from build123d import *

# Parameters (mm, degrees)
SKETCH1_W           = 128.5875
SKETCH1_H           = 111.125
BOSS_EXTRUDE1_DEPTH = 3.175
SKETCH2_R           = 22.356171926
SKETCH2_R_2         = 6.377074628
SKETCH2_R_3         = 4.503964563
CUT_EXTRUDE1_DEPTH  = 0.508
SKETCH4_R           = 2.446965281
SKETCH4_R_2         = 2.441870248
SKETCH4_R_3         = 1.365573368
SKETCH4_R_4         = 1.359710966
SKETCH4_W           = 6.35
SKETCH4_H           = 2.432656747
SKETCH4_H_2         = 2.571304572
SKETCH4_H_3         = 2.507941143
SKETCH4_H_4         = 2.659157088
CUT_EXTRUDE11_DEPTH = 1.5875


with BuildPart() as part:
    # Sketch1 → Boss-Extrude1 (new body)
    with BuildSketch(Plane(origin=(0, 0, 0), x_dir=(1, 0, 0), z_dir=(0, 1, 0))):
        Rectangle(SKETCH1_W, SKETCH1_H)
    extrude(amount=BOSS_EXTRUDE1_DEPTH)

    # Sketch2 → Cut-Extrude1 (cut)
    # profile 1 of 4: a face of its own
    with BuildSketch(Plane(origin=(0, 3.175, 0), x_dir=(1, 0, 0), z_dir=(0, 1, 0))):
        with BuildLine():
            add(Edge.make_bspline(
                [(-40.987833639, 33.604755502), (-52.791869615, 51.393160856), (-34.670548488, 41.369579914)],
                knots=[0, 0, 0, 1, 1, 1], degree=2))
            ThreePointArc((-40.987833639, 33.604755502), (-38.269367043, 37.845284908), (-34.670548488, 41.369579914))
        make_face()
    # profile 2 of 4: a face of its own
    with BuildSketch(Plane(origin=(0, 3.175, 0), x_dir=(1, 0, 0), z_dir=(0, 1, 0))):
        with BuildLine():
            add(Edge.make_bspline(
                [(-7.184604133, 41.369579914), (7.863520936, 53.974007146), (-0.867318981, 33.604755502)],
                knots=[0, 0, 0, 1, 1, 1], degree=2))
            ThreePointArc((-7.184604133, 41.369579914), (-3.585785578, 37.845284908), (-0.867318981, 33.604755502))
        make_face()
    # profile 3 of 4: a face of its own
    with BuildSketch(Plane(origin=(0, 3.175, 0), x_dir=(1, 0, 0), z_dir=(0, 1, 0))):
        with Locations((-20.92757631, 23.736397022)):
            Circle(SKETCH2_R)
        with Locations(Location((-20.92757631, 17.39779757, 0), (0, 0, 270))):
            Circle(SKETCH2_R_2, mode=Mode.SUBTRACT)
        with Locations(Location((-30.749586512, 27.886542178, 0), (0, 0, 270))):
            Circle(SKETCH2_R_3, mode=Mode.SUBTRACT)
        with Locations(Location((-11.797256967, 27.886542178, 0), (0, 0, 270))):
            Circle(SKETCH2_R_3, mode=Mode.SUBTRACT)
        with BuildLine():
            ThreePointArc((-30.749586512, 9.317085534), (-21.427716956, 3.728530924), (-11.797256967, 8.766728526))
            Line((-11.797256967, 8.766728526), (-30.749586512, 9.317085534))
        make_face(mode=Mode.SUBTRACT)
    # profile 4 of 4: a face of its own
    with BuildSketch(Plane(origin=(0, 3.175, 0), x_dir=(1, 0, 0), z_dir=(0, 1, 0))):
        with BuildLine():
            Line((-11.466221212, -23.168163392), (-10.968659983, -38.249198381))
            Line((-10.968659983, -38.249198381), (-4.570137716, -38.249198381))
            Line((-4.570137716, -38.249198381), (-4.570137716, -29.496558138))
            ThreePointArc((-4.570137716, -29.496558138), (-3.428830963, -30.22282284), (-2.256517086, -30.897894461))
            Line((-2.256517086, -30.897894461), (-1.884638787, -42.169491419))
            Line((-1.884638787, -42.169491419), (4.518768835, -42.169491419))
            Line((4.518768835, -42.169491419), (4.518768835, -33.609716863))
            ThreePointArc((4.518768835, -33.609716863), (14.659430985, -34.563354284), (24.550701184, -32.133286996))
            Line((24.550701184, -32.133286996), (24.780651804, -39.103069122))
            Line((24.780651804, -39.103069122), (31.179561384, -39.103069122))
            Line((31.179561384, -39.103069122), (31.179561384, -28.20870534))
            ThreePointArc((31.179561384, -28.20870534), (32.167865558, -27.406768429), (33.121940536, -26.564397437))
            Line((33.121940536, -26.564397437), (33.604851579, -41.201386667))
            Line((33.604851579, -41.201386667), (40.008784891, -41.201386667))
            Line((40.008784891, -41.201386667), (40.008784891, -17.235252664))
            ThreePointArc((40.008784891, -17.235252664), (34.852114754, 16.699623637), (1.416829228, 24.461630995))
            ThreePointArc((1.416829228, 24.461630995), (1.425653826, 24.099061731), (1.428595616, 23.736397022))
            ThreePointArc((1.428595616, 23.736397022), (-3.993475132, 9.140690788), (-17.629643976, 1.624814864))
            ThreePointArc((-17.629643976, 1.624814864), (-17.261411086, -11.446232799), (-11.466221212, -23.168163392))
        make_face()
    extrude(amount=-CUT_EXTRUDE1_DEPTH, mode=Mode.SUBTRACT)

    # Sketch4 → Cut-Extrude11 (cut)
    with BuildSketch(Plane(origin=(0, 3.175, 0), x_dir=(1, 0, 0), z_dir=(0, 1, 0))):
        with Locations(Location((-30.774197511, 25.825339041, 0), (0, 0, 270))):
            Circle(SKETCH4_R)
        with Locations(Location((-11.798514882, 25.825339041, 0), (0, 0, 270))):
            Circle(SKETCH4_R_2)
        with Locations(Location((-18.425247422, 17.392416095, 0), (0, 0, 270))):
            Circle(SKETCH4_R_3)
        with Locations(Location((-23.55125419, 17.392416095, 0), (0, 0, 270))):
            Circle(SKETCH4_R_4)
        with Locations((-7.793659983, -39.465526755)):
            Rectangle(SKETCH4_W, SKETCH4_H)
        with Locations((1.290361213, -43.455143705)):
            Rectangle(SKETCH4_W, SKETCH4_H_2)
        with Locations((27.955651804, -40.357039693)):
            Rectangle(SKETCH4_W, SKETCH4_H_3)
        with Locations((36.779851579, -42.530965211)):
            Rectangle(SKETCH4_W, SKETCH4_H_4)
    extrude(amount=-CUT_EXTRUDE11_DEPTH, mode=Mode.SUBTRACT)


solid = part.part
The model under review builds one solid part; all positions refer to its coordinate system, in mm. A direction names the side the tool comes from. Coordinates: 2 decimals unless noted, no trailing zeros. Write each loop counter-clockwise with the first axis right and the second up, starting at its lowest first coordinate (ties: lowest second). Pieces come first, ordered by that corner, then holes. Notation, with made-up numbers: (63.25, -8) - (70.25, -8) arc R4 cw to (70.25, -4) - close; hole circle Ø3 at (-26, -24). An arc over 180 degrees is marked (long way). Answer as a JSON object with one key per item and string values. Group by question number.
1. Add section C-C (z = 21). Give the boundary of the cut face in (x, y) (3 decimals).
2. Add section B-B (x = 36.5). Give the boundary of the cut face in (y, z) (1 decimal), plus the area to 3 significant figures.
3. Machinability: for faces 1 (the face through (-20.72, 2.92, -46.09)), 2 (the face through (-1, 0, -1)), which of the approach directions +Z, -Z, +X, -X, +Y, -Y give a long, thin tool a straight path to every point of the face, cutting with its end or side? Answer none if there is none.
4. Add section A-A (z = 3). Give the boundary of the cut face in (x, y) (3 decimals).
5. To check wall thickness, follow probe 1 along X at (y, z) = (2.45, 42.5); probe 2 along Y at (x, z) = (0, -21); probe 3 along Z at (x, y) = (-19.5, 1.75). State the ranges of each line that lie inside material, in increasing order.
6. Clearance check with a flat-ended pin moving along its axis: pin 1 Ø4.5 at (x, z) = (-30.77, -25.83) entering from +Y. State where the tip first meets the part, or that it passes through.
7. Mouldability with a two-part tool opening along Z and no side actions: class faces 3 (the face through (-21.587, 2.925, -3.734)), 4 (the face through (-12, 3.175, -29)), 5 (the face through (-1, 2, -55.562)) as pulls with the +Z half, pulls with the -Z half, needs draft (parallel to the pull), parting line crosses it, or undercut.
Findings:
{
 "1": {"outline": "(-64.294, 0) - (64.294, 0) - (64.294, 3.175) - (40.009, 3.175) - (40.009, 2.667) - (-13.049, 2.667) - (-13.049, 3.175) - (-64.294, 3.175) - close"},
 "2": {"outline": "(0, -55.6) - (3.2, -55.6) - (3.2, -14.8) - (2.7, -14.8) - (2.7, 41.2) - (1.6, 41.2) - (1.6, 43.9) - (3.2, 43.9) - (3.2, 55.6) - (0, 55.6) - close", "area": "320 mm²"},
 "3": {"face 1": "+Y", "face 2": "+Z, -Z, +X, -X, -Y"},
 "4": {"outline": "(-64.294, 0) - (64.294, 0) - (64.294, 3.175) - (42.97, 3.175) - (42.97, 2.667) - (-18.146, 2.667) - (-18.146, 3.175) - (-64.294, 3.175) - close"},
 "5": {"probe 1": "-64.29 to -1.88, 4.47 to 33.6, 39.95 to 64.29", "probe 2": "0 to 2.67", "probe 3": "-55.56 to -18.23, -16.55 to 55.56"},
 "6": {"pin 1": "y = 1.59"},
 "7": {"face 3": "undercut", "face 4": "needs draft", "face 5": "pulls with the -Z half"}
}
